```python
from build123d import *

# Parameters (mm, degrees)
SKETCH1_W           = 50
SKETCH1_H           = 100
BOSS_EXTRUDE1_DEPTH = 5
SKETCH2_W           = 52.895350152
SKETCH2_H           = 9.9
CUT_EXTRUDE1_DEPTH  = 6
FILLET1_R           = 5
SKETCH3_W           = 30.5
SKETCH3_H           = 30.5
CUT_EXTRUDE2_DEPTH  = 6


with BuildPart() as part:
    # Sketch1 → Boss-Extrude1 (new body)
    with BuildSketch(Plane(origin=(0, 0, 0), x_dir=(1, 0, 0), z_dir=(0, 1, 0))):
        Rectangle(SKETCH1_W, SKETCH1_H)
    extrude(amount=BOSS_EXTRUDE1_DEPTH)

    # Sketch2 → Cut-Extrude1 (cut, through all)
    with BuildSketch(Plane(origin=(0, 5, 0), x_dir=(1, 0, 0), z_dir=(0, 1, 0))):
        with Locations((5.447675076, -34.01)):
            Rectangle(SKETCH2_W, SKETCH2_H)
    cut_extrude1 = extrude(amount=-CUT_EXTRUDE1_DEPTH, mode=Mode.SUBTRACT)

    # Mirror1: Cut-Extrude1 across plane
    add(cut_extrude1.mirror(Plane.XY), mode=Mode.SUBTRACT)

    # Fillet1
    fillet1_edges = [part.edges().sort_by_distance(p)[0] for p in [
        (25, 2.5, 38.96),
        (25, 2.5, 29.06),
        (25, 2.5, -29.06),
        (25, 2.5, -38.96),
        (25, 2.5, 50),
        (-25, 2.5, 50),
        (-25, 2.5, -50),
        (25, 2.5, -50),
    ]]
    fillet(fillet1_edges, radius=FILLET1_R)

    # Sketch3 → Cut-Extrude2 (cut, through all)
    with BuildSketch(Plane(origin=(0, 5, 0), x_dir=(1, 0, 0), z_dir=(0, 1, 0))):
        Rectangle(SKETCH3_W, SKETCH3_H)
    extrude(amount=-CUT_EXTRUDE2_DEPTH, mode=Mode.SUBTRACT)


solid = part.part
```
Geometry: final body of the model. Coordinates: model frame, mm. A direction names the side the tool comes from. Round coordinates to 2 decimals unless told otherwise and drop trailing zeros. Loops run counter-clockwise (first coordinate to the right, second up) from the corner with the lowest first, then second, coordinate; pieces in that order, holes last. Notation, with made-up numbers: (48, -6) -> (76, -6) arc R19 ccw to (76, 15) -> close; hole circle Ø11 at (10, -20.75). An arc over 180 degrees is marked (long way). Use one line per item in the form item = value.
Item 1: Material intervals for probe 1 along Z at (x, y) = (-0.5, 0.8); probe 2 along Z at (x, y) = (16, 4.35); probe 3 along X at (y, z) = (4.4, -7), sorted ascending.
Evaluation:
probe_1 = -50 to -38.96, -29.06 to -15.25, 15.25 to 29.06, 38.96 to 50
probe_2 = -50 to -38.96, -29.06 to 29.06, 38.96 to 50
probe_3 = -25 to -15.25, 15.25 to 25
Item 2: Access query for faces 1 (the flat face through (0, 3, -15.25)), 2 (the flat face through (-1, 3, 29.06)), 3 (the flat face through (-25, 2, 1)). Directions: +Z, -Z, +X, -X, +Y, -Y. A direction counts if a zero-diameter tool reaches every point of the face in a straight line with its end or side. Return the directions, or none.
Evaluation:
face_1 = +Y, -Y
face_2 = +X, +Y, -Y
face_3 = +Z, -Z, -X, +Y, -Y
Item 3: Cut plane A-A on x = 14. Output: boundary loops of the cut face in (y, z).
Evaluation:
outline = (0, -50) -> (5, -50) -> (5, -38.96) -> (0, -38.96) -> close; (0, -29.06) -> (5, -29.06) -> (5, -15.25) -> (0, -15.25) -> close; (0, 15.25) -> (5, 15.25) -> (5, 29.06) -> (0, 29.06) -> close; (0, 38.96) -> (5, 38.96) -> (5, 50) -> (0, 50) -> close
Item 4: Contact query for a flat-ended pin moving along its axis: pin 1 Ø2 at (y, z) = (2, 32.5) entering from +X. Output: stop coordinate, or through.
Evaluation:
pin_1 = -21
Item 5: Draft query along Z for faces 4 (the flat face through (25, 2, 0)), 5 (the cylindrical face through (23, 3, -49)), 6 (the flat face through (15.25, 3, 0)). Return one class per face: released by +Z, released by -Z, zero draft, split by the parting line, or undercut.
Evaluation:
face_4 = zero draft
face_5 = released by -Z
face_6 = undercut
Item 6: Cut plane D-D on z = 28. Output: boundary loops of the cut face in (x, y).
Evaluation:
outline = (-25, 0) -> (23.08, 0) -> (23.08, 5) -> (-25, 5) -> close
Item 7: Cut plane C-C on z = -5.5. Output: boundary loops of the cut face in (x, y).
Evaluation:
outline = (-25, 0) -> (-15.25, 0) -> (-15.25, 5) -> (-25, 5) -> close; (15.25, 0) -> (25, 0) -> (25, 5) -> (15.25, 5) -> close
Item 8: Cut plane B-B on y = 0.95. Output: boundary loops of the cut face in (x, z), then the cut area to 3 significant figures.
Evaluation:
outline = (-25, -45) arc R5 ccw to (-20, -50) -> (20, -50) arc R5 ccw to (25, -45) -> (25, -43.96) arc R5 ccw to (20, -38.96) -> (-21, -38.96) -> (-21, -29.06) -> (20, -29.06) arc R5 ccw to (25, -24.06) -> (25, 24.06) arc R5 ccw to (20, 29.06) -> (-21, 29.06) -> (-21, 38.96) -> (20, 38.96) arc R5 ccw to (25, 43.96) -> (25, 45) arc R5 ccw to (20, 50) -> (-20, 50) arc R5 ccw to (-25, 45) -> close; hole (-15.25, -15.25) -> (15.25, -15.25) -> (15.25, 15.25) -> (-15.25, 15.25) -> close
area = 3,120 mm2
